from build123d import *

# Parameters (mm, degrees)
SKETCH2_R           = 2
SKETCH2_R_2         = 10
BOSS_EXTRUDE6_DEPTH = 5
CUT_EXTRUDE9_DEPTH  = 10


with BuildPart() as part:
    # Sketch2 → Boss-Extrude6 (new body)
    with BuildSketch(Plane.XY):
        with BuildLine():
            Line((-130.703145502, -382.314175973), (-100.703145502, -382.314175973))
            Line((-100.703145502, -382.314175973), (-45.95440816, -327.565438631))
            Line((-45.95440816, -327.565438631), (-45.95440816, -297.565438631))
            Line((-45.95440816, -297.565438631), (233.296854498, -297.565438631))
            Line((233.296854498, -297.565438631), (233.296854498, -409.565438631))
            ThreePointArc((233.296854498, -409.565438631), (226.225786687, -412.494370819), (223.296854498, -419.565438631))
            Line((223.296854498, -419.565438631), (223.296854498, -499.565438631))
            ThreePointArc((223.296854498, -499.565438631), (226.225786687, -506.636506443), (233.296854498, -509.565438631))
            Line((233.296854498, -509.565438631), (233.296854498, -621.565438631))
            Line((233.296854498, -621.565438631), (-45.95440816, -621.565438631))
            Line((-45.95440816, -621.565438631), (-45.95440816, -591.565438631))
            Line((-45.95440816, -591.565438631), (-100.703145502, -536.81670129))
            Line((-100.703145502, -536.81670129), (-130.703145502, -536.81670129))
            Line((-130.703145502, -536.81670129), (-130.703145502, -382.314175973))
        make_face()
        with Locations((15.633601358, -331.79452168)):
            Circle(SKETCH2_R, mode=Mode.SUBTRACT)
        with Locations((-14.366398642, -361.79452168)):
            Circle(SKETCH2_R, mode=Mode.SUBTRACT)
        with Locations((15.633601358, -391.79452168)):
            Circle(SKETCH2_R, mode=Mode.SUBTRACT)
        with Locations((45.633601358, -361.79452168)):
            Circle(SKETCH2_R, mode=Mode.SUBTRACT)
        with Locations((15.633601358, -361.79452168)):
            Circle(SKETCH2_R_2, mode=Mode.SUBTRACT)
        with Locations((-24.366398642, -401.79452168)):
            Circle(SKETCH2_R_2, mode=Mode.SUBTRACT)
        with BuildLine():
            Line((-29.596250394, -304.524677965), (-26.596250394, -304.524677965))
            ThreePointArc((-26.596250394, -304.524677965), (-23.596250394, -307.524677965), (-26.596250394, -310.524677965))
            Line((-26.596250394, -310.524677965), (-29.596250394, -310.524677965))
            ThreePointArc((-29.596250394, -310.524677965), (-32.596250394, -307.524677965), (-29.596250394, -304.524677965))
        make_face(mode=Mode.SUBTRACT)
        with BuildLine():
            Line((-114.203145502, -429.565438631), (-114.203145502, -489.565438631))
            ThreePointArc((-114.203145502, -489.565438631), (-120.703145502, -496.065438631), (-127.203145502, -489.565438631))
            Line((-127.203145502, -489.565438631), (-127.203145502, -429.565438631))
            ThreePointArc((-127.203145502, -429.565438631), (-120.703145502, -423.065438631), (-114.203145502, -429.565438631))
        make_face(mode=Mode.SUBTRACT)
        with BuildLine():
            Line((216.938696732, -304.524677965), (213.938696732, -304.524677965))
            ThreePointArc((213.938696732, -304.524677965), (210.938696732, -307.524677965), (213.938696732, -310.524677965))
            Line((213.938696732, -310.524677965), (216.938696732, -310.524677965))
            ThreePointArc((216.938696732, -310.524677965), (219.938696732, -307.524677965), (216.938696732, -304.524677965))
        make_face(mode=Mode.SUBTRACT)
        with BuildLine():
            Line((216.938696732, -614.606199297), (213.938696732, -614.606199297))
            ThreePointArc((213.938696732, -614.606199297), (210.938696732, -611.606199297), (213.938696732, -608.606199297))
            Line((213.938696732, -608.606199297), (216.938696732, -608.606199297))
            ThreePointArc((216.938696732, -608.606199297), (219.938696732, -611.606199297), (216.938696732, -614.606199297))
        make_face(mode=Mode.SUBTRACT)
        with BuildLine():
            Line((-29.596250394, -614.606199297), (-26.596250394, -614.606199297))
            ThreePointArc((-26.596250394, -614.606199297), (-23.596250394, -611.606199297), (-26.596250394, -608.606199297))
            Line((-26.596250394, -608.606199297), (-29.596250394, -608.606199297))
            ThreePointArc((-29.596250394, -608.606199297), (-32.596250394, -611.606199297), (-29.596250394, -614.606199297))
        make_face(mode=Mode.SUBTRACT)
        with BuildLine():
            Line((-117.703145502, -395.473744081), (-117.703145502, -398.473744081))
            ThreePointArc((-117.703145502, -398.473744081), (-120.703145502, -401.473744081), (-123.703145502, -398.473744081))
            Line((-123.703145502, -398.473744081), (-123.703145502, -395.473744081))
            ThreePointArc((-123.703145502, -395.473744081), (-120.703145502, -392.473744081), (-117.703145502, -395.473744081))
        make_face(mode=Mode.SUBTRACT)
        with BuildLine():
            Line((53.671223169, -301.453147058), (133.671223169, -301.453147058))
            ThreePointArc((133.671223169, -301.453147058), (139.742754077, -307.524677965), (133.671223169, -313.596208873))
            Line((133.671223169, -313.596208873), (53.671223169, -313.596208873))
            ThreePointArc((53.671223169, -313.596208873), (47.599692262, -307.524677965), (53.671223169, -301.453147058))
        make_face(mode=Mode.SUBTRACT)
        with BuildLine():
            Line((-117.703145502, -523.657133181), (-117.703145502, -520.657133181))
            ThreePointArc((-117.703145502, -520.657133181), (-120.703145502, -517.657133181), (-123.703145502, -520.657133181))
            Line((-123.703145502, -520.657133181), (-123.703145502, -523.657133181))
            ThreePointArc((-123.703145502, -523.657133181), (-120.703145502, -526.657133181), (-117.703145502, -523.657133181))
        make_face(mode=Mode.SUBTRACT)
        with BuildLine():
            Line((53.671223169, -617.677730205), (133.671223169, -617.677730205))
            ThreePointArc((133.671223169, -617.677730205), (139.742754077, -611.606199297), (133.671223169, -605.534668389))
            Line((133.671223169, -605.534668389), (53.671223169, -605.534668389))
            ThreePointArc((53.671223169, -605.534668389), (47.599692262, -611.606199297), (53.671223169, -617.677730205))
        make_face(mode=Mode.SUBTRACT)
    extrude(amount=BOSS_EXTRUDE6_DEPTH)

    # Sketch5 → Cut-Extrude9 (cut)
    with BuildSketch(Plane.XY.offset(5)):
        with BuildLine():
            Line((-130.703145502, -382.314175973), (-130.703145502, -536.81670129))
            Line((-130.703145502, -536.81670129), (-100.703145502, -536.81670129))
            Line((-100.703145502, -536.81670129), (-45.95440816, -591.565438631))
            Line((-45.95440816, -591.565438631), (-45.95440816, -621.565438631))
            Line((-45.95440816, -621.565438631), (233.296854498, -621.565438631))
            Line((233.296854498, -621.565438631), (233.296854498, -509.565438631))
            ThreePointArc((233.296854498, -509.565438631), (226.225786687, -506.636506443), (223.296854498, -499.565438631))
            Line((223.296854498, -499.565438631), (223.296854498, -419.565438631))
            ThreePointArc((223.296854498, -419.565438631), (226.225786687, -412.494370819), (233.296854498, -409.565438631))
            Line((233.296854498, -409.565438631), (233.296854498, -297.565438631))
            Line((233.296854498, -297.565438631), (-45.95440816, -297.565438631))
            Line((-45.95440816, -297.565438631), (-45.95440816, -327.565438631))
            Line((-45.95440816, -327.565438631), (-100.703145502, -382.314175973))
            Line((-100.703145502, -382.314175973), (-130.703145502, -382.314175973))
        make_face()
        with BuildLine():
            Line((-45.75440816, -327.648281344), (-100.620302789, -382.514175973))
            Line((-100.620302789, -382.514175973), (-130.503145502, -382.514175973))
            Line((-130.503145502, -382.514175973), (-130.503145502, -536.61670129))
            Line((-130.503145502, -536.61670129), (-100.620302789, -536.61670129))
            Line((-100.620302789, -536.61670129), (-45.75440816, -591.482595919))
            Line((-45.75440816, -591.482595919), (-45.75440816, -621.365438631))
            Line((-45.75440816, -621.365438631), (233.096854498, -621.365438631))
            Line((233.096854498, -621.365438631), (233.096854498, -509.763477658))
            ThreePointArc((233.096854498, -509.763477658), (226.013997916, -506.70686706), (223.096854498, -499.565438631))
            Line((223.096854498, -499.565438631), (223.096854498, -419.565438631))
            ThreePointArc((223.096854498, -419.565438631), (226.013997916, -412.424010203), (233.096854498, -409.367399604))
            Line((233.096854498, -409.367399604), (233.096854498, -297.765438631))
            Line((233.096854498, -297.765438631), (-45.75440816, -297.765438631))
            Line((-45.75440816, -297.765438631), (-45.75440816, -327.648281344))
        make_face(mode=Mode.SUBTRACT)
    extrude(amount=-CUT_EXTRUDE9_DEPTH, mode=Mode.SUBTRACT)


solid = part.part
Build history of the part. All positions in model axes, mm. A direction names the side the tool comes from. Round coordinates to 2 decimals unless told otherwise and drop trailing zeros. Write each loop counter-clockwise with the first axis right and the second up, starting at its lowest first coordinate (ties: lowest second). Pieces come first, ordered by that corner, then holes. Notation, with made-up numbers: M 26,-13.5 L 42,-13.5 A29 cw 42,7.5 Z; hole C 89.5,68.25 d6. An arc over 180 degrees is marked long. Answer as a JSON object with one key per item and string values. Group by question number.
(1) Cut at C-C (y = -323). Give the cut face in (x, z), and give its area (3 significant figures).
(2) Which spindle directions (+Z, -Z, +X, -X, +Y, -Y) get a long thin tool onto all of the face, cutting with end or side? Do faces 1 (the cylindrical face through (13.466, -371.557, 2.465)), 2 (the cylindrical face through (226.092, -506.786, 2.535)). Say none if no direction does.
(3) Cut at A-A (x = 76). Give the cut face in (y, z), and give its area (3 significant figures).
(4) Flat gauge pins, fed straight in: pin 1 (5 mm diameter, centred on x = 150.5, y = -488, fed in from -Z); pin 2 (2.5 mm diameter, centred on x = -122.5, z = 3, fed in from -Y); pin 3 (2.5 mm diameter, centred on y = -464.5, z = 3, fed in from +X). Where does each tip first touch, or does it go through?
(5) Mould opens along Y. For faces 3 (the cylindrical face through (-26.534, -411.557, 2.465)), 4 (the flat face through (54, -457, 5)), 5 (the flat face through (-72.803, -354.697, 2.535)) say: pulls with the +Y half, pulls with the -Y half, needs draft (parallel to the pull), parting line crosses it, or undercut.
(6) Cut at D-D (x = -59). Give the cut face in (y, z), and give its area (3 significant figures).
(7) Cut at B-B (y = -443). Give the cut face in (x, z).
(8) Drill centre lines: L1, parallel to Y at x = 84, z = 1.1; L2, parallel to X at y = -458, z = 4.85; L3, parallel to Y at x = -23, z = 4.1. Where is each one in solid material? Low to high.
Responses:
{
 "1": {"outline": "M -45.75,0 L 233.1,0 L 233.1,5 L -45.75,5 Z", "area": "1,390 mm2"},
 "2": {"face 1": "+Z, -Z", "face 2": "+Z, -Z, +X"},
 "3": {"outline": "M -621.37,0 L -617.68,0 L -617.68,5 L -621.37,5 Z; M -605.53,0 L -313.6,0 L -313.6,5 L -605.53,5 Z; M -301.45,0 L -297.77,0 L -297.77,5 L -301.45,5 Z", "area": "1,500 mm2"},
 "4": {"pin 1": "stops at z = 0", "pin 2": "stops at y = -536.62", "pin 3": "stops at x = 223.1"},
 "5": {"face 3": "undercut", "face 4": "needs draft", "face 5": "pulls with the +Y half"},
 "6": {"outline": "M -578.24,0 L -340.89,0 L -340.89,5 L -578.24,5 Z", "area": "1,190 mm2"},
 "7": {"outline": "M -130.5,0 L -127.2,0 L -127.2,5 L -130.5,5 Z; M -114.2,0 L 223.1,0 L 223.1,5 L -114.2,5 Z"},
 "8": {"L1": "y = -621.37 to -617.68, -605.53 to -313.6, -301.45 to -297.77", "L2": "x = -130.5 to -127.2, -114.2 to 223.1", "L3": "y = -621.37 to -411.7, -391.89 to -297.77"}
}
